from build123d import *

# Parameters (mm, degrees)
F2_DEPTH = 203.2
F3_DEPTH = 203.201
F4_R     = 14.7187970876
F5_DEPTH = 12.7


with BuildPart() as f2:
    # F0 (on Front) → F2 (new body)
    with BuildSketch(Plane.XZ):
        with BuildLine():
            Line((-76.2, 15.875), (-76.2, 0))
            Line((-76.2, 0), (-60.325, 0))
            ThreePointArc((-60.325, 0), (-64.9746798487, 11.2253201513), (-76.2, 15.875))
        make_face()
        with BuildLine():
            Line((-60.325, 0), (-76.2, 0))
            Line((-76.2, 0), (-76.2, -15.875))
            ThreePointArc((-76.2, -15.875), (-64.9746798487, -11.2253201513), (-60.325, 0))
        make_face()
        with BuildLine():
            Line((-76.2, -15.875), (-76.2, 0))
            Line((-76.2, 0), (-76.2, 15.875))
            ThreePointArc((-76.2, 15.875), (-92.075, 0), (-76.2, -15.875))
        make_face()
        with BuildLine():
            ThreePointArc((-76.2, 15.875), (-64.9746798487, 11.2253201513), (-60.325, 0))
            Line((-60.325, 0), (60.325, 0))
            ThreePointArc((60.325, 0), (64.9746798487, 11.2253201513), (76.2, 15.875))
            Line((76.2, 15.875), (-76.2, 15.875))
        make_face()
        with BuildLine():
            Line((60.325, 0), (-60.325, 0))
            ThreePointArc((-60.325, 0), (-64.9746798487, -11.2253201513), (-76.2, -15.875))
            Line((-76.2, -15.875), (76.2, -15.875))
            ThreePointArc((76.2, -15.875), (64.9746798487, -11.2253201513), (60.325, 0))
        make_face()
        with BuildLine():
            ThreePointArc((76.2, 15.875), (64.9746798487, 11.2253201513), (60.325, 0))
            Line((60.325, 0), (76.2, 0))
            Line((76.2, 0), (76.2, 15.875))
        make_face()
        with BuildLine():
            Line((76.2, 0), (60.325, 0))
            ThreePointArc((60.325, 0), (64.9746798487, -11.2253201513), (76.2, -15.875))
            Line((76.2, -15.875), (76.2, 0))
        make_face()
        with BuildLine():
            Line((76.2, 0), (76.2, -15.875))
            ThreePointArc((76.2, -15.875), (87.4253201513, -11.2253201513), (92.075, 0))
            ThreePointArc((92.075, 0), (87.4253201513, 11.2253201513), (76.2, 15.875))
            Line((76.2, 15.875), (76.2, 0))
        make_face()
    extrude(amount=F2_DEPTH)

    # F1 (on Front) → F3 (cut, through all)
    with BuildSketch(Plane.XZ):
        with BuildLine():
            ThreePointArc((76.2, -13.97), (62.23, 0), (76.2, 13.97))
            Line((76.2, 13.97), (-76.2, 13.97))
            ThreePointArc((-76.2, 13.97), (-66.3217182668, 9.8782817332), (-62.23, 0))
            ThreePointArc((-62.23, 0), (-66.3217182668, -9.8782817332), (-76.2, -13.97))
            Line((-76.2, -13.97), (76.2, -13.97))
        make_face()
        with BuildLine():
            ThreePointArc((90.17, 0), (86.0782817332, 9.8782817332), (76.2, 13.97))
            Line((76.2, 13.97), (76.2, -13.97))
            ThreePointArc((76.2, -13.97), (86.0782817332, -9.8782817332), (90.17, 0))
        make_face()
        with BuildLine():
            Line((76.2, -13.97), (76.2, 13.97))
            ThreePointArc((76.2, 13.97), (62.23, 0), (76.2, -13.97))
        make_face()
        with BuildLine():
            ThreePointArc((-62.23, 0), (-66.3217182668, 9.8782817332), (-76.2, 13.97))
            Line((-76.2, 13.97), (-76.2, -13.97))
            ThreePointArc((-76.2, -13.97), (-66.3217182668, -9.8782817332), (-62.23, 0))
        make_face()
        with BuildLine():
            Line((-76.2, -13.97), (-76.2, 13.97))
            ThreePointArc((-76.2, 13.97), (-90.17, 0), (-76.2, -13.97))
        make_face()
    extrude(amount=F3_DEPTH, mode=Mode.SUBTRACT)

    # F4 (on face) → F5 (cut)
    with BuildSketch(Plane.XY.offset(15.875)):
        with Locations((-38.1, -38.1)):
            Circle(F4_R)
    extrude(amount=-F5_DEPTH, mode=Mode.SUBTRACT)


solid = f2.part
Here's how the part is built. I have some questions about the finished solid (model axes, mm). A direction names the side the tool comes from. Round coordinates to 2 decimals unless told otherwise and drop trailing zeros. Loops run counter-clockwise (first coordinate to the right, second up) from the corner with the lowest first, then second, coordinate; pieces in that order, holes last.
1. We'd pull the mould along Z, two halves only. Please class faces 4 (the face through (1, -100, 15.875)), 5 (the face through (-90.167, -100.178, 0.307)), 6 (the face through (-0.4, -203.2, 14.2)): +Z half, -Z half, draft (parallel to the pull), parting line (faces both ways), or undercut.
Answer list:
face 4: +Z half
face 5: undercut
face 6: draft
2. If we section it at A-A on x = -38.1: Write out the boundary of the cut face in (y, z) (3 decimals).
Answer list:
outline: (-203.2, -15.875) - (0, -15.875) - (0, -13.97) - (-203.2, -13.97) - close; (-203.2, 13.97) - (-52.819, 13.97) - (-52.819, 15.875) - (-203.2, 15.875) - close; (-23.381, 13.97) - (0, 13.97) - (0, 15.875) - (-23.381, 15.875) - close
3. If I drill on line 1 along Z through (x, y) = (63, -193) (3 decimals); line 2 along X through (y, z) = (-94, -1); line 3 along Y through (x, z) = (-38.1, 14.7), over which ranges is the centre line in solid material (lowest first)?
Answer list:
line 1: z = -15.875 to -13.97, 13.97 to 15.875
line 2: x = -92.04 to -90.13, 90.13 to 92.04
line 3: y = -203.2 to -52.82, -23.38 to 0
4. If we section it at B-B on x = 43.5: Write out the boundary of the cut face in (y, z) (3 decimals).
Answer list:
outline: (-203.2, -15.875) - (0, -15.875) - (0, -13.97) - (-203.2, -13.97) - close; (-203.2, 13.97) - (0, 13.97) - (0, 15.875) - (-203.2, 15.875) - close
5. If we section it at D-D on z = -5: Write out the boundary of the cut face in (x, y), plus the area to 3 significant figures.
Answer list:
outline: (-91.27, -203.2) - (-89.24, -203.2) - (-89.24, 0) - (-91.27, 0) - close; (89.24, -203.2) - (91.27, -203.2) - (91.27, 0) - (89.24, 0) - close
area: 822 mm2
6. Which directions (+Z, -Z, +X, -X, +Y, -Y) give clear straight access to the entire face, cutting with the end or side of a thin tool? Please do faces 1 (the face through (1, -100, 13.97)), 2 (the face through (-0.4, 0, 14.2)), 3 (the face through (-41.29, -52.47, 14.94)).
Answer list:
face 1: +Y, -Y
face 2: +Z, -Z, +X, -X, +Y
face 3: +Z
7. For P1, Ø2, axis at y = -130, z = 7, coming from the +X side; P2, Ø10, axis at y = -88, z = -6.5, coming from the +X side; P3, Ø23.5, axis at x = -38.1, y = -38.1, coming from the +Z side, each with a flat end and sliding along its axis, tell me the tip position at first contact or that it passes through.
Answer list:
P1: stops at x = 90.9
P2: stops at x = 92
P3: stops at z = -13.97
8. If we section it at C-C on y = -64: Write out the boundary of the cut face in (x, z) (3 decimals), plus the area to 3 significant figures.
Answer list:
outline: (-76.2, -15.875) - (76.2, -15.875) arc R15.875 ccw to (76.2, 15.875) - (-76.2, 15.875) arc R15.875 ccw to start; hole (-76.2, -13.97) - (76.2, -13.97) arc R13.97 ccw to (76.2, 13.97) - (-76.2, 13.97) arc R13.97 ccw to start
area: 759 mm2
